Verification items for the finished model (mm, model axes). A direction names the side the tool comes from. Coordinates: 2 decimals unless noted, no trailing zeros. Loops run counter-clockwise (first coordinate to the right, second up) from the corner with the lowest first, then second, coordinate; pieces in that order, holes last. Notation, with made-up numbers: (-28.5, -9.5) - (-20.5, -9.5) arc R12 ccw to (-20.5, 8.5) - close; hole circle Ø4 at (35, 38). An arc over 180 degrees is marked (long way). Answer as CSV lines item,"result". Start each with the question number.
1. Cross-section at B-B (z = 1). Enter the section's corners in (x, y).
2. Gauge pin test, flat ends, axial feed: P1, Ø10.5, axis at x = -192.5, y = -134.5, coming from the +Z side; P2, Ø2.5, axis at y = -165.9, z = 67, coming from the +X side; P3, Ø2, axis at x = -195.4, y = -118.9, coming from the -Z side; P4, Ø6, axis at x = -203.5, y = -124, coming from the +Z side. Record the tip position at first contact, or that the pin passes through.
3. Set-up check for faces 5 (the flat face through (-196.9, -166, -60)), 6 (the flat face through (-213.9, -129, 67)), 7 (the flat face through (-198, -177.9, 0)): record each of +Z, -Z, +X, -X, +Y, -Y from which the full face is reachable in a straight line by a thin tool's end or side.
4. Release check for a two-part mould opening along Y. For faces 1 (the cylindrical face through (-209.87, -110.75, 68.99)), 2 (the flat face through (-204.4, -142.5, -54.5)), 3 (the flat face through (-194, -112.9, 3)), 4 (the flat face through (-200, -174, 62)) record: pulls with the +Y half, pulls with the -Y half, needs draft (parallel to the pull), parting line crosses it, or undercut.
5. Material ranges on line 1 (Y direction, x = -195, z = 6.5); line 2 (X direction, y = -173.85, z = -45); line 3 (X direction, y = -120.5, z = 45), recorded low to high. Write a range as [from, to].
6. Cross-section at A-A (z = -45). Enter the section's corners in (x, y), plus the area to 3 significant figures.
```python
from build123d import *

# Parameters (mm, degrees)
SKETCH165_W     = 75
SKETCH165_H     = 144
PAD045_DEPTH    = 10
FILLET025_R     = 10
CHAMFER010_SIZE = 6
SKETCH166_R     = 2
POCKET056_DEPTH = 6
PAD046_DEPTH    = 20
SKETCH169_R     = 1.75
POCKET057_DEPTH = 5
CHAMFER011_SIZE = 7
SKETCH172_R     = 2
POCKET059_DEPTH = 5


with BuildPart() as part:
    # Sketch165 → Pad045 (new body)
    with BuildSketch(Plane.YZ):
        with Locations((5.5, 0)):
            Rectangle(SKETCH165_W, SKETCH165_H)
    extrude(amount=PAD045_DEPTH)

    # Fillet025
    fillet025_edges = [part.edges().sort_by_distance(p)[0] for p in [
        (5, 43, -72),
        (5, -32, -72),
        (5, -32, 72),
        (5, 43, 72),
    ]]
    fillet(fillet025_edges, radius=FILLET025_R)

    # Chamfer010
    chamfer010_edges = [part.edges().sort_by_distance(p)[0] for p in [
        (0, 5.5, 72),
        (0, -32, 0),
        (0, 43, 0),
        (0, 5.5, -72),
    ]]
    chamfer(chamfer010_edges, length=CHAMFER010_SIZE)

    # Sketch166 (on Face4 of Chamfer010) → Pocket056 (cut)
    with BuildSketch(Plane.YZ.offset(10)):
        with Locations((-15, 67)):
            Circle(SKETCH166_R)
        with Locations((22, 67)):
            Circle(SKETCH166_R)
    extrude(amount=-POCKET056_DEPTH, mode=Mode.SUBTRACT)

    # Sketch167 (on Face4 of Pocket056) → Pad046 (join)
    with BuildSketch(Plane.YZ.offset(10)):
        Polygon((-27, 62), (-27, -63), (43, -63), (43, 62), (38, 62), (38, -58), (-22, -58), (-22, 62), align=None)
    extrude(amount=PAD046_DEPTH)

    # Sketch169 (on Face13 of Pad046) → Pocket057 (cut)
    with BuildSketch(Plane(origin=(0, 0, -58), x_dir=(0, -1, 0), z_dir=(0, 0, 1))):
        with Locations((-32, 22.5)):
            Circle(SKETCH169_R)
        with BuildLine():
            ThreePointArc((12, 24), (10.5, 22.5), (12, 21))
            Line((12, 21), (19, 21))
            ThreePointArc((19, 21), (20.5, 22.5), (19, 24))
            Line((12, 24), (19, 24))
        make_face()
    extrude(amount=-POCKET057_DEPTH, mode=Mode.SUBTRACT)

    # Chamfer011
    chamfer011_edges = [part.edges().sort_by_distance(p)[0] for p in [
        (10, 8, -58),
        (10, -22, 2),
        (10, 38, 2),
    ]]
    chamfer(chamfer011_edges, length=CHAMFER011_SIZE)

    # Sketch172 (on Face18 of Chamfer011) → Pocket059 (cut)
    with BuildSketch(Plane.ZX.offset(-22)):
        with Locations((-45, 25)):
            Circle(SKETCH172_R)
    extrude(amount=-POCKET059_DEPTH, mode=Mode.SUBTRACT)


with BuildPart() as part_1:
    # Body016 placement: moved
    add(part.part.moved(Location((-217.9, -150.9, 0))))


solid = part_1.part
```
Values follow:
1,outline,"(-217.9, -176.9) - (-211.9, -182.9) - (-207.9, -182.9) - (-207.9, -177.9) - (-187.9, -177.9) - (-187.9, -172.9) - (-200.9, -172.9) - (-207.9, -165.9) - (-207.9, -119.9) - (-200.9, -112.9) - (-187.9, -112.9) - (-187.9, -107.9) - (-211.9, -107.9) - (-217.9, -113.9) - close"
2,P1,"stops at z = -58"
2,P2,"stops at x = -213.9"
2,P3,"passes through"
2,P4,"stops at z = -52.4"
3,face 5,"+Z, -Z"
3,face 6,"+X"
3,face 7,"+Z, -Z, +X, -Y"
4,face 1,"pulls with the +Y half"
4,face 2,"undercut"
4,face 3,"undercut"
4,face 4,"needs draft"
5,line 1,"y = [-177.9, -172.9], [-112.9, -107.9]"
5,line 2,"x = [-217.9, -194.9], [-190.9, -187.9]"
5,line 3,"x = [-217.9, -207.9]"
6,outline,"(-217.9, -176.9) - (-211.9, -182.9) - (-207.9, -182.9) - (-207.9, -177.9) - (-194.9, -177.9) - (-194.9, -172.9) - (-200.9, -172.9) - (-207.9, -165.9) - (-207.9, -119.9) - (-200.9, -112.9) - (-187.9, -112.9) - (-187.9, -107.9) - (-211.9, -107.9) - (-217.9, -113.9) - close; (-190.9, -177.9) - (-187.9, -177.9) - (-187.9, -172.9) - (-190.9, -172.9) - close"
6,area,"943 mm²"
